Build history of the part. All positions in model axes, mm. Face numbers are marked on the shaded views. A direction names the side the tool comes from. Coordinates: 2 decimals unless noted, no trailing zeros. Order: outer loops, then holes, each group sorted by start corner. A loop starts at its lowest first (then second) coordinate and runs counter-clockwise, first axis right, second up. Notation, with made-up numbers: (83.25, 11.25) - (90.25, 11.25) arc R17 ccw to (90.25, 21.25) - close; hole circle Ø8 at (51.5, 17.5). An arc over 180 degrees is marked (long way). One line per item, written item: value.
from build123d import *

# Parameters (mm, degrees)
SKETCH1_W           = 20.25
SKETCH1_H           = 9
BOSS_EXTRUDE1_DEPTH = 9.1
SKETCH2_W           = 18.65
SKETCH2_H           = 7.4
CUT_EXTRUDE1_DEPTH  = 7.1
SKETCH2_3_W         = 0.8
SKETCH2_3_H         = 0.8
BOSS_EXTRUDE2_DEPTH = 12.5
SKETCH3_W           = 4.5
SKETCH3_H           = 7.1
CUT_EXTRUDE2_DEPTH  = 2.1
SKETCH5_W           = 4.5
SKETCH5_H           = 6.4
CUT_EXTRUDE3_DEPTH  = 0.8
SKETCH6_W           = 4.5
SKETCH6_H           = 6.4
CUT_EXTRUDE4_DEPTH  = 0.8
SKETCH8_W           = 3.34
SKETCH8_H           = 2
CUT_EXTRUDE5_DEPTH  = 35.242661924


with BuildPart() as part:
    # Sketch1 → Boss-Extrude1 (new body)
    with BuildSketch(Plane(origin=(0, 0, 0), x_dir=(1, 0, 0), z_dir=(0, 1, 0))):
        with Locations((-29.615572658, 24.590099186)):
            Rectangle(SKETCH1_W, SKETCH1_H)
    extrude(amount=BOSS_EXTRUDE1_DEPTH)

    # Sketch2 → Cut-Extrude1 (cut)
    with BuildSketch(Plane(origin=(0, 9.1, 0), x_dir=(1, 0, 0), z_dir=(0, 1, 0))):
        with Locations((-29.615572658, 24.590099186)):
            Rectangle(SKETCH2_W, SKETCH2_H)
    extrude(amount=-CUT_EXTRUDE1_DEPTH, mode=Mode.SUBTRACT)

    # Sketch2<3> → Boss-Extrude2 (add)
    with BuildSketch(Plane(origin=(0, 9.1, 0), x_dir=(1, 0, 0), z_dir=(0, 1, 0))):
        with Locations((-32.155572658, 23.320099186)):
            Rectangle(SKETCH2_3_W, SKETCH2_3_H)
        with Locations((-29.615572658, 23.320099186)):
            Rectangle(SKETCH2_3_W, SKETCH2_3_H)
        with Locations((-27.075572658, 23.320099186)):
            Rectangle(SKETCH2_3_W, SKETCH2_3_H)
        with Locations((-24.535572658, 23.320099186)):
            Rectangle(SKETCH2_3_W, SKETCH2_3_H)
        with Locations((-29.615572658, 25.860099186)):
            Rectangle(SKETCH2_3_W, SKETCH2_3_H)
        with Locations((-27.075572658, 25.860099186)):
            Rectangle(SKETCH2_3_W, SKETCH2_3_H)
        with Locations((-24.535572658, 25.860099186)):
            Rectangle(SKETCH2_3_W, SKETCH2_3_H)
        with Locations((-32.155572658, 25.860099186)):
            Rectangle(SKETCH2_3_W, SKETCH2_3_H)
        with Locations((-34.695572658, 23.320099186)):
            Rectangle(SKETCH2_3_W, SKETCH2_3_H)
        with Locations((-34.695572658, 25.860099186)):
            Rectangle(SKETCH2_3_W, SKETCH2_3_H)
    extrude(amount=-BOSS_EXTRUDE2_DEPTH)

    # Sketch3 → Cut-Extrude2 (cut)
    with BuildSketch(Plane.XY.offset(-20.090099186)):
        with Locations((-29.615572658, 5.55)):
            Rectangle(SKETCH3_W, SKETCH3_H)
    extrude(amount=-CUT_EXTRUDE2_DEPTH, mode=Mode.SUBTRACT)

    # Sketch5 → Cut-Extrude3 (cut)
    with BuildSketch(Plane.ZY.offset(39.740572658)):
        with Locations((-24.590099186, 3.2)):
            Rectangle(SKETCH5_W, SKETCH5_H)
    extrude(amount=-CUT_EXTRUDE3_DEPTH, mode=Mode.SUBTRACT)

    # Sketch6 → Cut-Extrude4 (cut)
    with BuildSketch(Plane(origin=(-19.490572658, 0, 0), x_dir=(0, 0, -1), z_dir=(1, 0, 0))):
        with Locations((24.590099186, 3.2)):
            Rectangle(SKETCH6_W, SKETCH6_H)
    extrude(amount=-CUT_EXTRUDE4_DEPTH, mode=Mode.SUBTRACT)

    # Sketch8 → Cut-Extrude5 (cut, through all)
    with BuildSketch(Plane.ZY.offset(35.095572658)):
        with Locations((-24.590099186, -2.4)):
            Rectangle(SKETCH8_W, SKETCH8_H)
    extrude(amount=-CUT_EXTRUDE5_DEPTH, mode=Mode.SUBTRACT)


solid = part.part
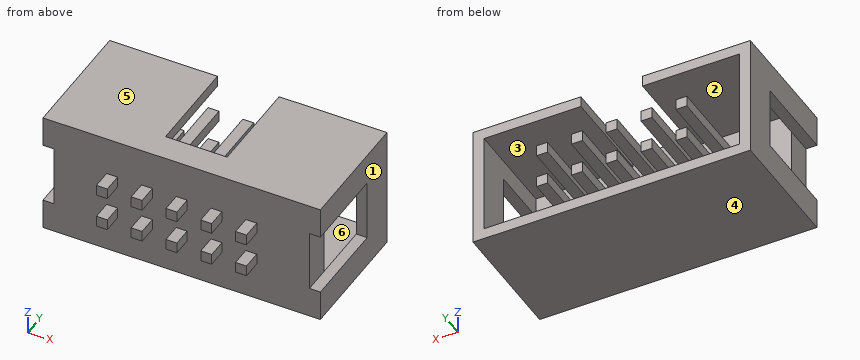
1. Band-saw the part on C-C, the plane z = -21.75. Give the cut face in (x, y).
Values found:
outline: (-39.74, 0) - (-19.49, 0) - (-19.49, 9.1) - (-20.29, 9.1) - (-20.29, 2) - (-38.94, 2) - (-38.94, 9.1) - (-39.74, 9.1) - close
2. Band-saw the part on D-D, the plane y = 2.5. Count the separate pieces of the cut face and the enclosed holes in it, and give its area (3 significant figures).
Values found:
separate pieces: 13
enclosed holes: 0
area: 39.8 mm2
3. Flat gauge pins, fed straight in: P1, Ø0.6, axis at y = -0.5, z = -23, coming from the +X side; P2, Ø0.6, axis at x = -34.5, y = -1, coming from the -Z side; P3, Ø0.9, axis at y = 4, z = -23.5, coming from the -X side; P4, Ø5, axis at x = -34.5, z = -27, coming from the -Y side. Where does each tip first touch, or does it go through?
Values found:
P1: stops at x = -24.14
P2: stops at z = -26.26
P3: stops at x = -35.1
P4: stops at y = -1.4
4. Band-saw the part on B-B, the plane x = -24.5. Give the cut face in (y, z), and give its area (3 significant figures).
Values found:
outline: (-1.4, -26.26) - (0, -26.26) - (0, -29.09) - (9.1, -29.09) - (9.1, -28.29) - (2, -28.29) - (2, -26.26) - (9.1, -26.26) - (9.1, -25.46) - (2, -25.46) - (2, -23.72) - (9.1, -23.72) - (9.1, -22.92) - (2, -22.92) - (2, -20.89) - (9.1, -20.89) - (9.1, -20.09) - (0, -20.09) - (0, -22.92) - (-1.4, -22.92) - (-1.4, -23.72) - (0, -23.72) - (0, -25.46) - (-1.4, -25.46) - close
area: 43.0 mm2
5. Two-plate mould, pull along Z, no slides. Class the marked faces 1, 2, 3 and 4: pulls with the +Z half, pulls with the -Z half, needs draft (parallel to the pull), parting line crosses it, or undercut.
Values found:
face 1: needs draft
face 2: undercut
face 3: undercut
face 4: pulls with the -Z half
6. 3-axis set-ups, long thin cutter, end or side, ignore diameter. For the marked faces 5 and 6: which of +Z, -Z, +X, -X, +Y, -Y reach the whole face in a straight line?
Values found:
face 5: +Z, +X, -X, +Y, -Y
face 6: +Y
7. Probe line 1 along Z through (x, y) = (-32.5, 2.25); line 2 along X through (y, z) = (6, -23.5); line 3 along Z through (x, y) = (-22.5, 3.5). List the from-to ranges inside material, lowest first.
Values found:
line 1: z = -29.09 to -28.29, -26.26 to -25.46, -23.72 to -22.92, -20.89 to -20.09
line 2: x = -35.1 to -34.3, -32.56 to -31.76, -30.02 to -29.22, -27.48 to -26.68, -24.94 to -24.14
line 3: z = -29.09 to -28.29, -20.89 to -20.09
8. Band-saw the part on A-A, the plane z = -25. Give the cut face in (x, y).
Values found:
outline: (-39.74, 6.4) - (-38.94, 6.4) - (-38.94, 9.1) - (-39.74, 9.1) - close; (-38.94, 0) - (-20.29, 0) - (-20.29, 2) - (-38.94, 2) - close; (-20.29, 6.4) - (-19.49, 6.4) - (-19.49, 9.1) - (-20.29, 9.1) - close
